Part model, mm, in its own coordinate system. A direction names the side the tool comes from. Round coordinates to 2 decimals unless told otherwise and drop trailing zeros. Write each loop counter-clockwise with the first axis right and the second up, starting at its lowest first coordinate (ties: lowest second). Pieces come first, ordered by that corner, then holes. Notation, with made-up numbers: (56.25, -37.75) -> (62.25, -37.75) arc R15 cw to (62.25, -22.75) -> close; hole circle Ø8 at (68, -6). An arc over 180 degrees is marked (long way). Return JSON: item names as keys, results as strings. Group by question number.
```python
from build123d import *

# Parameters (mm, degrees)
BOSS_EXTRUDE1_DEPTH      = 8.001
BOSS_EXTRUDE1_DEPTH_BACK = 8.001
CUT_EXTRUDE1_DEPTH       = 8.001
CUT_EXTRUDE2_DEPTH       = 8.001
SKETCH5_R                = 2.5
CUT_EXTRUDE3_DEPTH       = 10
SKETCH6_R                = 2.5
CUT_EXTRUDE4_DEPTH       = 10
CHAMFER1_SIZE            = 1


with BuildPart() as part:
    # Sketch2 → Boss-Extrude1 (new body, two sides)
    with BuildSketch(Plane(origin=(0, 0, 0), x_dir=(0, 0, -1), z_dir=(1, 0, 0))) as boss_extrude1_sk:
        Polygon((-20.07, 0), (0, 0), (0, -20.07), (-2, -20.07), (-2, -2), (-20.07, -2), align=None)
    extrude(amount=BOSS_EXTRUDE1_DEPTH)
    extrude(boss_extrude1_sk.sketch, amount=-BOSS_EXTRUDE1_DEPTH_BACK)

    # Sketch3 → Cut-Extrude1 (cut)
    with BuildSketch(Plane.XZ.offset(2)):
        with BuildLine():
            Line((-8.001, 12.069), (-12.725932728, 12.069))
            Line((-12.725932728, 12.069), (-12.725932728, 24.915681473))
            Line((-12.725932728, 24.915681473), (12.141962569, 24.915681473))
            Line((12.141962569, 24.915681473), (12.141962569, 12.069))
            Line((12.141962569, 12.069), (8.001, 12.069))
            ThreePointArc((8.001, 12.069), (0, 20.07), (-8.001, 12.069))
        make_face()
    extrude(amount=-CUT_EXTRUDE1_DEPTH, mode=Mode.SUBTRACT)

    # Sketch4 → Cut-Extrude2 (cut)
    with BuildSketch(Plane.XY.offset(2)):
        with BuildLine():
            Line((-8.001, -12.069), (-10.480924408, -12.069))
            Line((-10.480924408, -12.069), (-10.480924408, -22.641723191))
            Line((-10.480924408, -22.641723191), (9.892967081, -22.641723191))
            Line((9.892967081, -22.641723191), (9.892967081, -12.069))
            Line((9.892967081, -12.069), (8.001, -12.069))
            ThreePointArc((8.001, -12.069), (0, -20.07), (-8.001, -12.069))
        make_face()
    extrude(amount=-CUT_EXTRUDE2_DEPTH, mode=Mode.SUBTRACT)

    # Sketch5 → Cut-Extrude3 (cut)
    with BuildSketch(Plane.XY.offset(2)):
        with Locations((0, -12.069)):
            Circle(SKETCH5_R)
    extrude(amount=-CUT_EXTRUDE3_DEPTH, mode=Mode.SUBTRACT)

    # Sketch6 → Cut-Extrude4 (cut)
    with BuildSketch(Plane.XZ.offset(2)):
        with Locations((0, 12.069)):
            Circle(SKETCH6_R)
    extrude(amount=-CUT_EXTRUDE4_DEPTH, mode=Mode.SUBTRACT)

    # Chamfer1
    chamfer1_edges = [part.edges().sort_by_distance(p)[0] for p in [
        (-2.5, -12.069, 2),
        (-2.5, -2, 12.069),
    ]]
    chamfer(chamfer1_edges, length=CHAMFER1_SIZE)


solid = part.part
```
Item 1: Cut at D-D (y = -7.5). Write the cut outline in (x, z), then the cut area to 3 significant figures.
Item 2: Two-plate mould, pull along Y, no slides. Class faces 1 (the face through (0, 0, 8)), 2 (the face through (0.176, -1.014, 20.068)), 3 (the face through (0.176, -20.068, 1.014)), 4 (the face through (-0.33, -9.59, 0.51)): released by +Y, released by -Y, zero draft, split by the parting line, or undercut.
Item 3: Flat gauge pins, fed straight in: P1, Ø1.5, axis at x = -2.5, y = -18, coming from the +Z side; P2, Ø10, axis at y = -8, z = 9, coming from the +X side. Where does each tip first touch, or does it go through?
Item 4: Wall check: L1, parallel to Y at x = 0, z = 0.45; L2, parallel to Z at x = 0, y = -0.65; L3, parallel to Z at x = -5.25, y = -10.5. Give the ranges that are in metal, low to high.
Item 5: Cut at C-C (x = 6.5). Write the cut outline in (y, z), then the cut area to 3 significant figures.
Item 6: Cut at A-A (x = 0). Write the cut outline in (y, z), then the cut area to 3 significant figures.
Item 7: Which spindle directions (+Z, -Z, +X, -X, +Y, -Y) get a long thin tool onto all of the face, cutting with end or side? Do faces 5 (the face through (0, -8, 0)), 6 (the face through (0, -7, 2)). Say none if no direction does.
Item 8: Cut at B-B (z = 3.5). Write the cut outline in (x, y).
Checks:
{
 "1": {"outline": "(-8, 0) -> (8, 0) -> (8, 2) -> (-8, 2) -> close", "area": "32.0 mm2"},
 "2": {"face 1": "released by +Y", "face 2": "zero draft", "face 3": "released by -Y", "face 4": "undercut"},
 "3": {"P1": "stops at z = 2", "P2": "passes through"},
 "4": {"L1": "y = -20.07 to -14.57, -9.57 to 0", "L2": "z = 0 to 9.57, 14.57 to 20.07", "L3": "z = 0 to 2"},
 "5": {"outline": "(-16.73, 0) -> (0, 0) -> (0, 16.73) -> (-2, 16.73) -> (-2, 2) -> (-16.73, 2) -> close", "area": "62.9 mm2"},
 "6": {"outline": "(-20.07, 0) -> (-14.57, 0) -> (-14.57, 1) -> (-15.57, 2) -> (-20.07, 2) -> close; (-9.57, 0) -> (0, 0) -> (0, 9.57) -> (-1, 9.57) -> (-2, 8.57) -> (-2, 2) -> (-8.57, 2) -> (-9.57, 1) -> close; (-2, 15.57) -> (-1, 14.57) -> (0, 14.57) -> (0, 20.07) -> (-2, 20.07) -> close", "area": "54.3 mm2"},
 "7": {"face 5": "-Z, +X, -X, +Y, -Y", "face 6": "+Z, +X, -X, -Y"},
 "8": {"outline": "(-8, -2) -> (8, -2) -> (8, 0) -> (-8, 0) -> close"}
}
